Model file for the job. Use its own axes, mm. A direction names the side the tool comes from. Coordinates: 2 decimals unless noted, no trailing zeros. Write each loop counter-clockwise with the first axis right and the second up, starting at its lowest first coordinate (ties: lowest second). Pieces come first, ordered by that corner, then holes.
Q1. Which spindle directions (+Z, -Z, +X, -X, +Y, -Y) get a long thin tool onto all of the face, cutting with end or side? Do faces 4 (the cylindrical face through (3.78, 12.89, -27.86)), 5 (the cylindrical face through (10.321, 49.427, -79.643)), 6 (the flat face through (1.96, 24.94, -44.09)). Say none if no direction does.
Q2. Band-saw the part on D-D, the plane y = 20.5. Write the cut outline in (x, z).
Q3. Drill centre lines: probe 1 along Y at (x, z) = (16.55, -27.5); probe 2 along X at (y, z) = (19, -39.5); probe 3 along X at (y, z) = (41, -53). Where is each one in solid material? Low to high.
Q4. Pin check, flat tips, straight feed: P1, Ø1.5, axis at x = 19.5, z = -42.5, coming from the -Y side; P2, Ø15.5, axis at x = 12.5, y = 19.5, coming from the -Z side; P3, Ø5, axis at x = 29.5, z = -26, coming from the -Y side; P4, Ø5.5, axis at y = 41, z = -45, coming from the -X side. Stop position of each tip, or through.
Q5. Band-saw the part on C-C, the plane y = 33.5. Write the cut outline in (x, z), plus the area to 3 significant figures.
Q6. Pull direction Y, two halves, no side cores. Call faces 1 (the flat face through (27.5, 41.5, -56.52)), 2 (the flat face through (32.14, 24.9, -9.86)), 3 (the flat face through (31.8, 31.1, -20)): released by +Y, released by -Y, zero draft, split by the parting line, or undercut.
Q7. Band-saw the part on B-B, the plane x = 16.55. Write the cut outline in (y, z).
Autodesk Inventor part; units mm, degrees
ref_plane "YZ Plane" through (0, 0, 0) normal (1, 0, 0) x (0, 1, 0)
ref_plane "XZ Plane" through (0, 0, 0) normal (0, 1, 0) x (-1, 0, 0)
ref_plane "XY Plane" through (0, 0, 0) normal (0, 0, 1) x (1, 0, 0)
sketch "Sketch1" plane through (0, 0, 0) normal (0, 0, 1) x (1, 0, 0)
  line L0 (0, 0) -> (33.1, 0)
  line L1 (33.1, 0) -> (33.1, 54)
  line L2 (33.1, 54) -> (0, 54)
  line L3 (0, 54) -> (0, 0)
  arc A0 (32.9068, 34.9287) -> (0.1932, 34.9287) centre (16.55, 37.45) ccw
  line L4 (0, 37.45) -> (1.95, 12)
  line L5 (1.95, 12) -> (13.9851, 12) construction
  line L6 (8.2338, 0) -> (24.8662, 0)
  line L7 (33.1, 37.45) -> (31.15, 12)
  arc A1 (1.95, 12) -> (8.2338, 0) centre (16.55, 12) ccw
  arc A2 (24.8662, 0) -> (31.15, 12) centre (16.55, 12) ccw
  dimension "d0" = 33.1
  dimension "d1" = 54
  dimension "d2" = 33.1
extrude "Extrusion1" add sketch "Sketch1" against normal blind 67.52 contours A1 L4 A0 L7 A2 L0
sketch "Sketch3" plane through (0, 0, 0) normal (0, 0, 1) x (1, 0, 0)
  arc A0 (33.1, 37.45) -> (0, 37.45) centre (16.55, 37.45) ccw
  circle A1 centre (16.55, 37.45) radius 13.5
  arc A2 (24.8662, 0) -> (31.15, 12) centre (16.55, 12) ccw
  line L0 (8.817, 1.8) -> (24.283, 1.8)
  line L1 (8.817, 1.8) -> (24.283, 1.8) construction
  line L2 (10.0048, 23) -> (23.0952, 23)
  arc A3 (10.0048, 23) -> (8.817, 1.8) centre (16.55, 12) ccw
  arc A4 (24.283, 1.8) -> (23.0952, 23) centre (16.55, 12) ccw
  point P0 (0, 0)
  dimension "d7" = 27
extrude "Extrusion2" cut sketch "Sketch3" against normal blind 56.52
sketch "Sketch4" plane through (0, 0, -67.52) normal (0, 0, -1) x (-1, 0, 0)
  arc A0 (0, 37.45) -> (-33.1, 37.45) centre (-16.55, 37.45) ccw
  circle A1 centre (-16.55, 37.45) radius 13.5
  point P0 (0, 0)
extrude "Extrusion3" add sketch "Sketch4" along normal blind 24.59
sketch "Sketch7" plane through (0, 0, -67.52) normal (0, 0, -1) x (-1, 0, 0)
  circle A0 centre (-16.55, 37.45) radius 13.5
  arc A1 (0, 37.45) -> (-33.1, 37.45) centre (-16.55, 37.45) ccw
  arc A2 (-23.0952, 23) -> (-24.283, 1.8) centre (-16.55, 12) ccw
  line L0 (-1.95, 12) -> (0, 37.45)
  line L1 (-24.8662, 0) -> (-8.2338, 0)
  line L2 (-24.8662, 0) -> (-8.2338, 0)
  arc A3 (-8.2338, 0) -> (-1.95, 12) centre (-16.55, 12) ccw
  arc A4 (-31.15, 12) -> (-24.8662, 0) centre (-16.55, 12) ccw
  arc A5 (-31.15, 12) -> (-24.8662, 0) centre (-16.55, 12) ccw
  line L3 (-31.15, 12) -> (-33.1, 37.45)
  arc A6 (-1, 37.4877) -> (-32.1, 37.45) centre (-16.55, 37.45) ccw
  line L4 (-1, 37.4877) -> (-2.9501, 12.0376)
  arc A7 (-8.5525, 1) -> (-2.9501, 12.0376) centre (-16.55, 12) ccw
  line L5 (-8.5525, 1) -> (-24.5475, 1)
  arc A8 (-30.1499, 12.0376) -> (-24.5475, 1) centre (-16.55, 12) ccw
  line L6 (-30.1499, 12.0376) -> (-32.1029, 37.5264)
  point P0 (0, 0)
  point P1 (-32.1, 37.4877)
  dimension "d21" = 1
extrude "Extrusion6" cut sketch "Sketch7" against normal blind 47.52 contours L0 A3 L1 A4 L3 A1
sketch "Sketch8" plane through (16.55, 37.45, -92.11) normal (0, 0, -1) x (-1, 0, 0)
  circle A0 centre (0, 0) radius 11.5
  point P0 (16.55, -37.45)
  dimension "d24" = 23
extrude "Extrusion7" cut sketch "Sketch8" against normal blind 44.77
sketch "Sketch11" plane through (0, 0, -67.52) normal (0, 0, -1) x (-1, 0, 0)
  arc A0 (0, 37.45) -> (-33.1, 37.45) centre (-16.55, 37.45) ccw
  line L0 (-33.1, 37.45) -> (-28.1, 37.45) construction
  line L1 (-33.1, 12.45) -> (-32.1, 12.45)
  line L2 (-32.1, 12.45) -> (-32.1, 42.45)
  line L3 (-32.1, 42.45) -> (-33.1, 42.45)
  line L4 (-33.1, 42.45) -> (-33.1, 12.45)
  point P0 (0, 0)
  dimension "d39" = 1
extrude "Extrusion9" add sketch "Sketch11" against normal blind 47.52
sketch "Sketch12" plane through (0, 0, -67.52) normal (0, 0, -1) x (-1, 0, 0)
  line L0 (-32.1, 12.45) -> (-33.1, 12.45)
  line L1 (-32.1, 42.45) -> (-32.1, 24.3987)
  line L2 (-33.1, 12.45) -> (-32.1, 12.45)
  line L3 (-32.1, 12.45) -> (-32.1, 42.45)
  line L4 (-32.1, 42.45) -> (-33.1, 42.45)
  line L5 (-33.1, 42.45) -> (-33.1, 12.45)
  point P0 (0, 0)
extrude "Extrusion10" cut sketch "Sketch12" against normal blind 10
properties part number "Big LRF Real"
Answer sheet:
1. face 4: +Z
1. face 5: -Z
1. face 6: -Z, -X, -Y
2. outline: (1.3, -20) - (2.3, -20) - (2.3, -67.52) - (30.8, -67.52) - (30.8, -20) - (31.8, -20) - (31.8, 0) - (26.12, 0) - (26.12, -56.52) - (6.98, -56.52) - (6.98, 0) - (1.3, 0) - close; (32.1, -57.52) - (33.1, -57.52) - (33.1, -20) - (32.1, -20) - close
3. probe 1: y = 1 to 1.8, 23 to 23.95, 50.95 to 53
3. probe 2: x = 2.42 to 5.83, 27.27 to 30.68, 32.1 to 33.1
3. probe 3: x = 1.41 to 3.53, 29.57 to 31.69, 32.1 to 33.1
4. P1: stops at y = 1
4. P2: stops at z = -92.11
4. P3: stops at y = 3.3
4. P4: stops at x = 1.02
5. outline: (0.3, -20) - (1.31, -20) - (1.31, -67.52) - (3.64, -67.52) - (3.64, -92.11) - (5.75, -92.11) - (5.75, -56.52) - (3.64, -56.52) - (3.64, 0) - (0.3, 0) - close; (27.35, -92.11) - (29.46, -92.11) - (29.46, -67.52) - (31.79, -67.52) - (31.79, -20) - (32.1, -20) - (32.1, -57.52) - (33.1, -57.52) - (33.1, -20) - (32.8, -20) - (32.8, 0) - (29.46, 0) - (29.46, -56.52) - (27.35, -56.52) - close
5. area: 543 mm2
6. face 1: undercut
6. face 2: released by -Y
6. face 3: zero draft
7. outline: (0, -20) - (1, -20) - (1, -67.52) - (23.95, -67.52) - (23.95, -92.11) - (25.95, -92.11) - (25.95, -56.52) - (23.95, -56.52) - (23.95, 0) - (23, 0) - (23, -56.52) - (1.8, -56.52) - (1.8, 0) - (0, 0) - close; (48.95, -92.11) - (50.95, -92.11) - (50.95, -67.52) - (53, -67.52) - (53, -20) - (54, -20) - (54, 0) - (50.95, 0) - (50.95, -56.52) - (48.95, -56.52) - close
